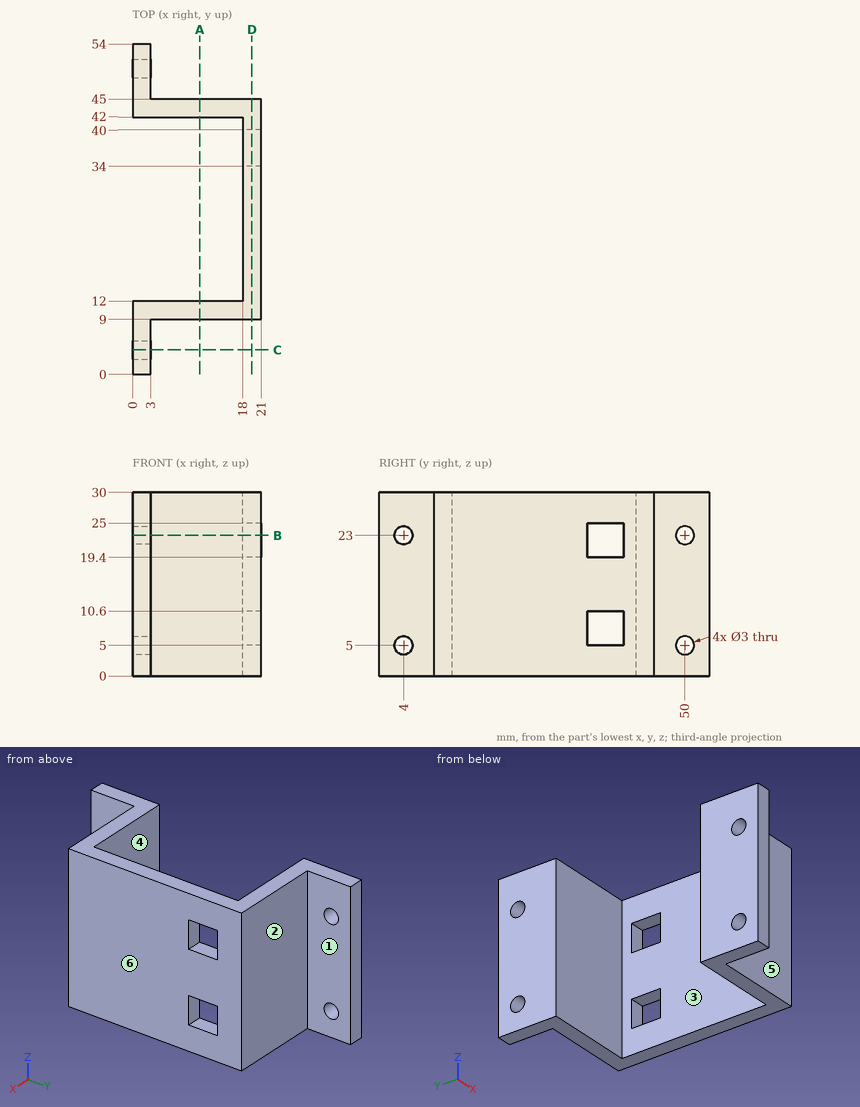
Drawing for the job (mm, zero at the part's lowest x, y, z). A direction names the side the tool comes from. Round coordinates to 2 decimals unless told otherwise and drop trailing zeros. Order: outer loops, then holes, each group sorted by start corner. A loop starts at its lowest first (then second) coordinate and runs counter-clockwise, first axis right, second up. Notation, with made-up numbers: (-3.5, 39.25) -> (55.5, 39.25) arc R14 cw to (55.5, 58.25) -> close; hole circle Ø4 at (62, 36.25). An arc over 180 degrees is marked (long way). Write item = value, one per line. Start each with the question number.
(1) Pin check, flat tips, straight feed: P1, Ø9, axis at y = 22.5, z = 18.5, coming from the -X side; P2, Ø2.5, axis at y = 50, z = 5, coming from the -X side; P3, Ø5.5, axis at x = 11, z = 8, coming from the +Y side; P4, Ø10, axis at x = 15.5, z = 6.5, coming from the -Y side. Stop position of each tip, or through.
(2) Probe line 1 (Y direction, x = 1.75, z = 23); line 2 (Z direction, x = 1.3, y = 4); line 3 (Y direction, x = 16, z = 17). List the from-to ranges inside material, lowest first. Write a range as [from, to].
(3) Cut at D-D, the plane x = 19.5. List the corners of the cut face in (y, z), then the cut area to 3 significant figures.
(4) Cut at A-A, the plane x = 11. List the corners of the cut face in (y, z), then the cut area to 3 significant figures.
(5) Pull direction Y, two halves, no side cores. Call the marked faces 1, 2 and 3: released by +Y, released by -Y, zero draft, split by the parting line, or undercut.
(6) Which spindle directions (+Z, -Z, +X, -X, +Y, -Y) get a long thin tool onto all of the face, cutting with end or side? Do the marked faces 4, 5 and 6. Say none if no direction does.
(7) Cut at B-B, the plane z = 23. List the corners of the cut face in (x, y), then the cut area to 3 significant figures.
(8) Cut at C-C, the plane y = 4. List the corners of the cut face in (x, z), then the cut area to 3 significant figures.
Model answer:
q1.P1 = 18
q1.P2 = through
q1.P3 = 45
q1.P4 = 9
q2.line_1 = [0, 2.5], [5.5, 12], [42, 48.5], [51.5, 54]
q2.line_2 = [0, 3.5], [6.5, 21.5], [24.5, 30]
q2.line_3 = [9, 12], [42, 45]
q3.outline = (9, 0) -> (45, 0) -> (45, 30) -> (9, 30) -> close; hole (34, 5) -> (40, 5) -> (40, 10.6) -> (34, 10.6) -> close; hole (34, 19.4) -> (40, 19.4) -> (40, 25) -> (34, 25) -> close
q3.area = 1,010 mm2
q4.outline = (9, 0) -> (12, 0) -> (12, 30) -> (9, 30) -> close; (42, 0) -> (45, 0) -> (45, 30) -> (42, 30) -> close
q4.area = 180 mm2
q5.face_1 = zero draft
q5.face_2 = released by +Y
q5.face_3 = undercut
q6.face_4 = +Z, -Z, -X
q6.face_5 = +Z, -Z, +X, -Y
q6.face_6 = +Z, -Z, +X, +Y, -Y
q7.outline = (0, 0) -> (3, 0) -> (3, 2.5) -> (0, 2.5) -> close; (0, 5.5) -> (3, 5.5) -> (3, 9) -> (21, 9) -> (21, 34) -> (18, 34) -> (18, 12) -> (0, 12) -> close; (0, 42) -> (18, 42) -> (18, 40) -> (21, 40) -> (21, 45) -> (3, 45) -> (3, 48.5) -> (0, 48.5) -> close; (0, 51.5) -> (3, 51.5) -> (3, 54) -> (0, 54) -> close
q7.area = 234 mm2
q8.outline = (0, 0) -> (3, 0) -> (3, 3.5) -> (0, 3.5) -> close; (0, 6.5) -> (3, 6.5) -> (3, 21.5) -> (0, 21.5) -> close; (0, 24.5) -> (3, 24.5) -> (3, 30) -> (0, 30) -> close
q8.area = 72.0 mm2
